Check sheet for the modelled part. Datum: model origin and axes. Units: mm. Face numbers are marked on the shaded views. A direction names the side the tool comes from. Round coordinates to 2 decimals unless told otherwise and drop trailing zeros. Write each loop counter-clockwise with the first axis right and the second up, starting at its lowest first coordinate (ties: lowest second). Pieces come first, ordered by that corner, then holes. Notation, with made-up numbers: M 70.25,54 L 96.25,54 A26 cw 96.25,87 Z; hole C 25.5,52 d3. An arc over 180 degrees is marked long. Put each result on its own line as item: value.
```python
from build123d import *
from build123d.topology import SkipClean

# Parameters (mm, degrees)
EXTRUDE_1_DEPTH             = 220
SKETCH_3_R                  = 1.55
SKETCH_3_R_2                = 2.1
CUT_EXTRUDE_1_DEPTH         = 10
SKETCH_6_R                  = 1.6
CUT_EXTRUDE_2_DEPTH         = 10
CHAMFER_1_SIZE              = 1
CHAMFER_1_SIZE2             = 0.707106781
SHEET_START                 = -114.419250373
SHEET_METAL_2_OUTLINE_W     = 220
SHEET_METAL_2_OUTLINE_H     = 86.5
SHEET_METAL_2_OUTLINE_R     = 1.55
SHEET_METAL_2_OUTLINE_R_2   = 2.1
SHEET_METAL_2_DEPTH         = 26.274603255
SHEET_START_2               = -87.816219993
SHEET_METAL_2_2_OUTLINE_W   = 220
SHEET_METAL_2_2_OUTLINE_H   = 87
SHEET_METAL_2_2_OUTLINE_R   = 1.55
SHEET_METAL_2_2_OUTLINE_R_2 = 2.1
SHEET_METAL_2_2_DEPTH       = 0.483052927
SHEET_START_3               = -89.230433555
SHEET_METAL_2_3_OUTLINE_W   = 220
SHEET_METAL_2_3_OUTLINE_H   = 0.5
SHEET_METAL_2_3_DEPTH       = 21.707106781
SHEET_METAL_2_4_DEPTH       = 220
SHEET_METAL_2_5_DEPTH       = 220
SHEET_START_4               = 44
SHEET_METAL_2_6_OUTLINE_R   = 1.6
SHEET_METAL_2_6_DEPTH       = 0.5
SKETCH_7_R                  = 1.75
CUT_EXTRUDE_3_DEPTH         = 10


with BuildPart() as part:
    # 草图2 → 凸台-拉伸1 (new body)
    with BuildSketch(Plane(origin=(0, 0, 0), x_dir=(1, 0, 0), z_dir=(0, 1, 0))):
        Polygon((-87.523326774, 42.5), (-112.419250373, 17.604076401), (-112.419250373, -17.604076401), (-87.523326774, -42.5), (-67.523326774, -42.5), (-67.523326774, -44), (-88.144647118, -44), (-113.919250373, -18.225396744), (-113.919250373, 18.225396744), (-89.644647118, 42.5), align=None)
    extrude(amount=EXTRUDE_1_DEPTH)

    # Sketch 3 → 切除-拉伸1 (cut)
    with BuildSketch(Plane.ZY.offset(113.919250373)):
        with Locations((-10, 5)):
            Circle(SKETCH_3_R)
        with Locations((10, 5)):
            Circle(SKETCH_3_R)
        with BuildLine():
            ThreePointArc((-8.45, 110), (-10, 111.55), (-11.55, 110))
            Line((-11.55, 110), (-8.45, 110))
        make_face()
        with BuildLine():
            Line((-8.45, 110), (-11.55, 110))
            ThreePointArc((-11.55, 110), (-10, 108.45), (-8.45, 110))
        make_face()
        with BuildLine():
            ThreePointArc((8.45, 110), (10, 108.45), (11.55, 110))
            Line((11.55, 110), (8.45, 110))
        make_face()
        with BuildLine():
            Line((8.45, 110), (11.55, 110))
            ThreePointArc((11.55, 110), (10, 111.55), (8.45, 110))
        make_face()
        with Locations((-10, 215)):
            Circle(SKETCH_3_R)
        with Locations((10, 215)):
            Circle(SKETCH_3_R)
        with Locations((0, 200)):
            Circle(SKETCH_3_R_2)
        with Locations((0, 165)):
            Circle(SKETCH_3_R_2)
        with Locations((0, 55)):
            Circle(SKETCH_3_R_2)
        with Locations((0, 20)):
            Circle(SKETCH_3_R_2)
    extrude(amount=-CUT_EXTRUDE_1_DEPTH, mode=Mode.SUBTRACT)

    # 草图6 → 切除-拉伸2 (cut)
    with BuildSketch(Plane.XY.offset(44)):
        with Locations((-76.693326774, 5)):
            Circle(SKETCH_6_R)
        with Locations((-76.693326774, 110)):
            Circle(SKETCH_6_R)
        with Locations((-76.693326774, 215)):
            Circle(SKETCH_6_R)
    extrude(amount=-CUT_EXTRUDE_2_DEPTH, mode=Mode.SUBTRACT)

    # 倒角1
    chamfer_1_edges = [part.edges().sort_by_distance(p)[0] for p in [
        (-87.523326774, 110, -42.5),
    ]]
    chamfer_1_side = [part.faces().sort_by_distance(p)[0] for p in [
        (-99.971288574, 110, -30.0520382),
    ]]
    chamfer(chamfer_1_edges, length=CHAMFER_1_SIZE, length2=CHAMFER_1_SIZE2, reference=chamfer_1_side[0])

    # Sheet Metal 2: read off the stored shape, not the designer's step
    # Sheet Metal 2 outline → Sheet Metal 2 (add)
    with SkipClean():  # the faces are left unmerged after this step: merging them gives an invalid solid
        with BuildSketch(Plane.YZ.offset(SHEET_START)):
            with Locations((110, 0.75)):
                Rectangle(SHEET_METAL_2_OUTLINE_W, SHEET_METAL_2_OUTLINE_H)
            with Locations((5, -10)):
                Circle(SHEET_METAL_2_OUTLINE_R, mode=Mode.SUBTRACT)
            with Locations((20, 0)):
                Circle(SHEET_METAL_2_OUTLINE_R_2, mode=Mode.SUBTRACT)
            with Locations((55, 0)):
                Circle(SHEET_METAL_2_OUTLINE_R_2, mode=Mode.SUBTRACT)
            with Locations((110, -10)):
                Circle(SHEET_METAL_2_OUTLINE_R, mode=Mode.SUBTRACT)
            with Locations((215, -10)):
                Circle(SHEET_METAL_2_OUTLINE_R, mode=Mode.SUBTRACT)
            with Locations((165, 0)):
                Circle(SHEET_METAL_2_OUTLINE_R_2, mode=Mode.SUBTRACT)
            with Locations((200, 0)):
                Circle(SHEET_METAL_2_OUTLINE_R_2, mode=Mode.SUBTRACT)
            with Locations((5, 10)):
                Circle(SHEET_METAL_2_OUTLINE_R, mode=Mode.SUBTRACT)
            with Locations((110, 10)):
                Circle(SHEET_METAL_2_OUTLINE_R, mode=Mode.SUBTRACT)
            with Locations((215, 10)):
                Circle(SHEET_METAL_2_OUTLINE_R, mode=Mode.SUBTRACT)
        extrude(amount=SHEET_METAL_2_DEPTH)

    # Sheet Metal 2 2 outline → Sheet Metal 2 2 (add)
    with SkipClean():  # the faces are left unmerged after this step: merging them gives an invalid solid
        with BuildSketch(Plane.YZ.offset(SHEET_START_2)):
            with Locations((110, 1)):
                Rectangle(SHEET_METAL_2_2_OUTLINE_W, SHEET_METAL_2_2_OUTLINE_H)
            with Locations((5, -10)):
                Circle(SHEET_METAL_2_2_OUTLINE_R, mode=Mode.SUBTRACT)
            with Locations((20, 0)):
                Circle(SHEET_METAL_2_2_OUTLINE_R_2, mode=Mode.SUBTRACT)
            with Locations((55, 0)):
                Circle(SHEET_METAL_2_2_OUTLINE_R_2, mode=Mode.SUBTRACT)
            with Locations((110, -10)):
                Circle(SHEET_METAL_2_2_OUTLINE_R, mode=Mode.SUBTRACT)
            with Locations((215, -10)):
                Circle(SHEET_METAL_2_2_OUTLINE_R, mode=Mode.SUBTRACT)
            with Locations((165, 0)):
                Circle(SHEET_METAL_2_2_OUTLINE_R_2, mode=Mode.SUBTRACT)
            with Locations((200, 0)):
                Circle(SHEET_METAL_2_2_OUTLINE_R_2, mode=Mode.SUBTRACT)
            with Locations((5, 10)):
                Circle(SHEET_METAL_2_2_OUTLINE_R, mode=Mode.SUBTRACT)
            with Locations((110, 10)):
                Circle(SHEET_METAL_2_2_OUTLINE_R, mode=Mode.SUBTRACT)
            with Locations((215, 10)):
                Circle(SHEET_METAL_2_2_OUTLINE_R, mode=Mode.SUBTRACT)
        extrude(amount=SHEET_METAL_2_2_DEPTH)

    # Sheet Metal 2 3 outline → Sheet Metal 2 3 (add)
    with SkipClean():  # the faces are left unmerged after this step: merging them gives an invalid solid
        with BuildSketch(Plane.YZ.offset(SHEET_START_3)):
            with Locations((110, 44.25)):
                Rectangle(SHEET_METAL_2_3_OUTLINE_W, SHEET_METAL_2_3_OUTLINE_H)
        extrude(amount=SHEET_METAL_2_3_DEPTH)

    # Sheet Metal 2 4 outline → Sheet Metal 2 4 (cut)
    with BuildSketch(Plane(origin=(0, 0, 0), x_dir=(1, 0, 0), z_dir=(0, 1, 0))):
        with BuildLine():
            Line((-87.816219993, 42.5), (-87.816219993, -42.207106781))
            ThreePointArc((-87.816219993, -42.207106781), (-87.593520149, -42.374842797), (-87.333167066, -42.474576765))
            Line((-87.333167066, -42.474576765), (-87.333167066, 42.5))
            Line((-87.333167066, 42.5), (-87.816219993, 42.5))
        make_face()
        with BuildLine():
            Line((-88.144647118, 42.5), (-88.937540337, 42.5))
            Line((-88.937540337, 42.5), (-88.230433555, 41.792893219))
            Line((-88.230433555, 41.792893219), (-112.126357154, 17.89696962))
            ThreePointArc((-112.126357154, 17.89696962), (-112.343129906, 17.572546271), (-112.419250373, 17.189862838))
            Line((-112.419250373, 17.189862838), (-112.419250373, -17.189862838))
            ThreePointArc((-112.419250373, -17.189862838), (-112.343129906, -17.572546271), (-112.126357154, -17.89696962))
            Line((-112.126357154, -17.89696962), (-88.144647118, -41.878679656))
            Line((-88.144647118, -41.878679656), (-88.144647118, 42.5))
        make_face()
        with BuildLine():
            ThreePointArc((-113.540570717, -19.311183182), (-114.190888971, -18.337913135), (-114.419250373, -17.189862838))
            Line((-114.419250373, -17.189862838), (-114.419250373, -44))
            Line((-114.419250373, -44), (-89.230433555, -44))
            Line((-89.230433555, -44), (-89.230433555, -44.5))
            Line((-89.230433555, -44.5), (-87.109113212, -44.5))
            ThreePointArc((-87.109113212, -44.5), (-88.257163509, -44.271638598), (-89.230433555, -43.621320344))
            Line((-89.230433555, -43.621320344), (-113.540570717, -19.311183182))
        make_face()
        with BuildLine():
            Line((-113.540570717, 19.311183182), (-90.351753899, 42.5))
            Line((-90.351753899, 42.5), (-114.419250373, 42.5))
            Line((-114.419250373, 42.5), (-114.419250373, 17.189862838))
            ThreePointArc((-114.419250373, 17.189862838), (-114.190888971, 18.337913135), (-113.540570717, 19.311183182))
        make_face()
    extrude(amount=SHEET_METAL_2_4_DEPTH, mode=Mode.SUBTRACT)

    # Sheet Metal 2 5 outline → Sheet Metal 2 5 (add)
    with BuildSketch(Plane(origin=(0, 0, 0), x_dir=(1, 0, 0), z_dir=(0, 1, 0))):
        with BuildLine():
            ThreePointArc((-87.109113212, -42.5), (-87.221859022, -42.493623864), (-87.333167066, -42.474576765))
            Line((-87.333167066, -42.474576765), (-87.333167066, -42.5))
            Line((-87.333167066, -42.5), (-87.109113212, -42.5))
        make_face()
        Polygon((-88.937540337, 42.5), (-89.644647118, 43.207106781), (-90.351753899, 42.5), align=None)
    extrude(amount=SHEET_METAL_2_5_DEPTH)

    # Sheet Metal 2 6 outline → Sheet Metal 2 6 (cut)
    with BuildSketch(Plane.XY.offset(SHEET_START_4)):
        with Locations((-76.693326774, 5)):
            Circle(SHEET_METAL_2_6_OUTLINE_R)
        with Locations((-76.693326774, 110)):
            Circle(SHEET_METAL_2_6_OUTLINE_R)
        with Locations((-76.693326774, 215)):
            Circle(SHEET_METAL_2_6_OUTLINE_R)
    extrude(amount=SHEET_METAL_2_6_DEPTH, mode=Mode.SUBTRACT)

    # 草图7 → 切除-拉伸3 (cut)
    with BuildSketch(Plane(origin=(-66.425876949, 0, -66.425876949), x_dir=(-0.7071067811865474, 0, 0.7071067811865477), z_dir=(-0.7071067811865477, 0, -0.7071067811865474))):
        with Locations((49.436299673, 215)):
            Circle(SKETCH_7_R)
        with Locations((49.436299673, 5)):
            Circle(SKETCH_7_R)
    extrude(amount=-CUT_EXTRUDE_3_DEPTH, mode=Mode.SUBTRACT)


solid = part.part
```
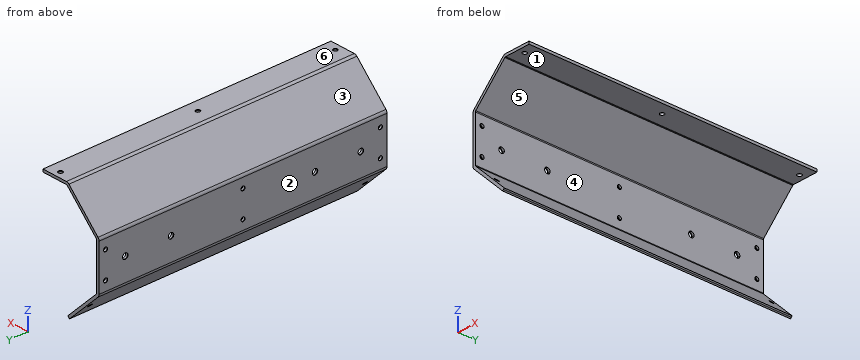
1. Access from +Z, -Z, +X, -X, +Y, -Y to the whole of each face (thin tool, end or side, straight path). Record for the marked faces 5 and 6.
Computed values:
face 5: +X, +Y, -Y
face 6: +Z, +X, -X, +Y, -Y
2. Release check for a two-part mould opening along Z. For the marked faces 1, 2, 3 and 4 record: +Z half, -Z half, draft (parallel to the pull), parting line (faces both ways), or undercut.
Computed values:
face 1: -Z half
face 2: draft
face 3: +Z half
face 4: undercut
3. Depth check by flat-ended pin: pin 1 Ø15.5 at (x, y) = (-75.5, 96.5) entering from -Z; pin 2 Ø5 at (x, y) = (-99.5, 104.5) entering from -Z; pin 3 Ø4 at (y, z) = (215, 10) entering from +X. Enter the tip coordinate at first touch or a pass-through.
Computed values:
pin 1: stops at z = 42.5
pin 2: stops at z = -35.85
pin 3: stops at x = -112.42
4. Cross-section at A-A (x = -110). Enter the section's corners in (y, z).
Computed values:
outline: M 0,-22.85 L 220,-22.85 L 220,-20.02 L 0,-20.02 Z; M 0,20.02 L 220,20.02 L 220,22.85 L 0,22.85 Z
5. Cross-section at B-B (y = 78). Enter the section's corners in (x, z), then the cut area to 3 significant figures.
Computed values:
outline: M -114.42,-17.19 A3 ccw -113.54,-19.31 L -89.64,-43.21 L -88.23,-41.79 L -112.13,-17.9 A1 cw -112.42,-17.19 L -112.42,17.19 A1 cw -112.13,17.9 L -87.82,42.21 A1 cw -87.11,42.5 L -67.52,42.5 L -67.52,44.5 L -87.11,44.5 A3 ccw -89.23,43.62 L -113.54,19.31 A3 ccw -114.42,17.19 Z
area: 254 mm2
6. Cross-section at D-D (x = -81). Enter the section's corners in (y, z).
Computed values:
outline: M 0,42.5 L 220,42.5 L 220,44.5 L 0,44.5 Z
7. Cross-section at C-C (z = 5.5). Enter the section's corners in (x, y), then the cut area to 3 significant figures.
Computed values:
outline: M -114.42,0 L -112.42,0 L -112.42,220 L -114.42,220 Z
area: 440 mm2
8. Scan lines: probe 1 along Y at (x, z) = (-114, 0); probe 2 along Y at (x, z) = (-114.2, 10); probe 3 along Z at (x, y) = (-100.5, 63). Record each from-to range of solid material in increasing order.
Computed values:
probe 1: y = 0 to 17.9, 22.1 to 52.9, 57.1 to 162.9, 167.1 to 197.9, 202.1 to 220
probe 2: y = 0 to 3.45, 6.55 to 108.45, 111.55 to 213.45, 216.55 to 220
probe 3: z = -32.35 to -29.52, 29.52 to 32.35
